Check sheet for the modelled part. Datum: model origin and axes. Units: mm. A direction names the side the tool comes from. Coordinates: 2 decimals unless noted, no trailing zeros. Loops run counter-clockwise (first coordinate to the right, second up) from the corner with the lowest first, then second, coordinate; pieces in that order, holes last. Notation, with made-up numbers: (-6.5, 50.25) -> (-2.5, 50.25) arc R27 ccw to (-2.5, 76.25) -> close; hole circle Ø5 at (7, 9.5). An arc over 180 degrees is marked (long way). Use one line per item in the form item = value.
from build123d import *

# Parameters (mm, degrees)
SKETCH_1_R          = 7.5
EXTRUDE_1_DEPTH     = 5
SKETCH_2_R          = 16.5
EXTRUDE_2_DEPTH     = 22.7
SKETCH_3_R          = 18.5
EXTRUDE_3_DEPTH     = 29
SKETCH_4_R          = 1.6
CUT_EXTRUDE_1_DEPTH = 10
SKETCH_5_R          = 6
EXTRUDE_4_DEPTH     = 6
SKETCH_6_R          = 3
EXTRUDE_5_DEPTH     = 15.5
CUT_EXTRUDE_START   = -12
CUT_EXTRUDE_2_DEPTH = 12
CHAMFER_1_SIZE      = 0.5
FILLET_1_R          = 1
FILLET_2_R          = 1
FILLET_3_R          = 1
SKETCH_8_R          = 0.654296706
EXTRUDE_6_DEPTH     = 4


with BuildPart() as part:
    # Эскиз1 → Бобышка-Вытянуть1 (new body)
    with BuildSketch(Plane(origin=(0, 0, 0), x_dir=(1, 0, 0), z_dir=(0, 1, 0))):
        with Locations(Location((0, 0, 0), (0, 0, 270))):
            Circle(SKETCH_1_R)
    extrude(amount=EXTRUDE_1_DEPTH)

    # Эскиз2 → Бобышка-Вытянуть2 (add)
    with BuildSketch(Plane(origin=(0, 5, 0), x_dir=(1, 0, 0), z_dir=(0, 1, 0))):
        with Locations(Location((0, 0, 0), (0, 0, 270))):
            Circle(SKETCH_2_R)
    extrude(amount=EXTRUDE_2_DEPTH)

    # Эскиз3 → Бобышка-Вытянуть3 (add)
    with BuildSketch(Plane(origin=(0, 27.7, 0), x_dir=(1, 0, 0), z_dir=(0, 1, 0))):
        with Locations(Location((0, 0, 0), (0, 0, 90))):
            Circle(SKETCH_3_R)
    extrude(amount=EXTRUDE_3_DEPTH)

    # Эскиз4 → Вырез-Вытянуть1 (cut)
    with BuildSketch(Plane(origin=(0, 56.7, 0), x_dir=(1, 0, 0), z_dir=(0, 1, 0))):
        with Locations(Location((0, -15.5, 0), (0, 0, 270))):
            Circle(SKETCH_4_R)
        with Locations(Location((-13.423393759, -7.75, 0), (0, 0, 270))):
            Circle(SKETCH_4_R)
        with Locations(Location((-13.423393759, 7.75, 0), (0, 0, 270))):
            Circle(SKETCH_4_R)
        with Locations(Location((0, 15.5, 0), (0, 0, 270))):
            Circle(SKETCH_4_R)
        with Locations(Location((13.423393759, 7.75, 0), (0, 0, 270))):
            Circle(SKETCH_4_R)
        with Locations(Location((13.423393759, -7.75, 0), (0, 0, 270))):
            Circle(SKETCH_4_R)
    extrude(amount=-CUT_EXTRUDE_1_DEPTH, mode=Mode.SUBTRACT)

    # Эскиз5 → Бобышка-Вытянуть4 (add)
    with BuildSketch(Plane(origin=(0, 56.7, 0), x_dir=(1, 0, 0), z_dir=(0, 1, 0))):
        with Locations(Location((-7, 0, 0), (0, 0, 270))):
            Circle(SKETCH_5_R)
    extrude(amount=EXTRUDE_4_DEPTH)

    # Эскиз6 → Бобышка-Вытянуть5 (add)
    with BuildSketch(Plane(origin=(0, 62.7, 0), x_dir=(1, 0, 0), z_dir=(0, 1, 0))):
        with Locations(Location((-7, 0, 0), (0, 0, 270))):
            Circle(SKETCH_6_R)
    extrude(amount=EXTRUDE_5_DEPTH)

    # Эскиз7 → Вырез-Вытянуть2 (cut)
    with BuildSketch(Plane(origin=(0, 78.2, 0), x_dir=(1, 0, 0), z_dir=(0, 1, 0)).offset(CUT_EXTRUDE_START)):
        with BuildLine():
            Line((-9.533328229, 1.606937486), (-9.465630062, -1.708996312))
            ThreePointArc((-9.465630062, -1.708996312), (-9.999374975, -0.061235296), (-9.533328229, 1.606937486))
        make_face()
    extrude(amount=CUT_EXTRUDE_2_DEPTH, mode=Mode.SUBTRACT)

    # Фаска1
    chamfer_1_edges = [part.edges().sort_by_distance(p)[0] for p in [
        (-4.371234847, 78.2, -1.445542725),
    ]]
    chamfer(chamfer_1_edges, length=CHAMFER_1_SIZE - 0.0001)  # a hair under: the kernel refuses the full size

    # Скругление1
    fillet_1_edges = [part.edges().sort_by_distance(p)[0] for p in [
        (0, 56.7, 18.5),
    ]]
    fillet(fillet_1_edges, radius=FILLET_1_R)

    # Скругление2
    fillet_2_edges = [part.edges().sort_by_distance(p)[0] for p in [
        (0, 27.7, -16.5),
    ]]
    fillet(fillet_2_edges, radius=FILLET_2_R)

    # Скругление3
    fillet_3_edges = [part.edges().sort_by_distance(p)[0] for p in [
        (0, 0, -7.5),
    ]]
    fillet(fillet_3_edges, radius=FILLET_3_R)

    # Эскиз8 → Бобышка-Вытянуть6 (add)
    with BuildSketch(Plane(origin=(0, 56.7, 0), x_dir=(1, 0, 0), z_dir=(0, 1, 0))):
        with Locations(Location((0, 0, 0), (0, 0, 270))):
            Circle(SKETCH_8_R)
    extrude(amount=EXTRUDE_6_DEPTH)


solid = part.part
(1) Scan lines: line 1 along X through (y, z) = (53.5, -7.75); line 2 along X through (y, z) = (50, -7); line 3 along Y through (x, z) = (-10.5, 7). Record each from-to range of solid material in increasing order.
Established:
line_1 = -16.8 to -15.02, -11.82 to 11.82, 15.02 to 16.8
line_2 = -17.12 to -14.84, -12.01 to 12.01, 14.84 to 17.12
line_3 = 5 to 56.7
(2) Go/stop test with flat-tipped pins: P1, Ø4, axis at x = 0, z = -15.5, coming from the +Y side; P2, Ø4, axis at y = 41.5, z = -7.5, coming from the +X side; P3, Ø8, axis at x = 14.5, z = -0.5, coming from the -Y side. Record where each tip stops, or that it passes through.
Established:
P1 = 56.7
P2 = 17.66
P3 = 5
(3) Tool access check on faces 1 (the cylindrical face through (0.07, 51.77, -17.1)), 2 (the cylindrical face through (-16.108, 15.698, -3.577)), 3 (the cylindrical face through (7.086, 41.504, -17.089)). Record the directions out of +Z, -Z, +X, -X, +Y, -Y that give a thin tool (end or side, any length) a straight path to the whole face; none if there is none.
Established:
face_1 = +Y
face_2 = -Y
face_3 = +Y, -Y
(4) Mould release check, pull along Z, two halves, no side actions. Record for faces 4 (the cylindrical face through (0.07, 51.77, 13.9)), 5 (the cylindrical face through (0.33, 2.972, -7.493)), 6 (the flat face through (0, 0, 0)): +Z half, -Z half, draft (parallel to the pull), parting line (faces both ways), or undercut.
Established:
face_4 = undercut
face_5 = parting line
face_6 = draft
(5) Section check A-A, the plane y = 51. Record the boundary of the cut face in (x, z), plus the area to 3 significant figures.
Established:
outline = circle Ø37 at (0, 0); hole circle Ø3.2 at (-13.42, -7.75); hole circle Ø3.2 at (-13.42, 7.75); hole circle Ø3.2 at (0, -15.5); hole circle Ø3.2 at (0, 15.5); hole circle Ø3.2 at (13.42, -7.75); hole circle Ø3.2 at (13.42, 7.75)
area = 1,030 mm²
